Autodesk Inventor part; units mm, degrees
ref_plane "YZ Plane" through (0, 0, 0) normal (1, 0, 0) x (0, 1, 0)
ref_plane "XZ Plane" through (0, 0, 0) normal (0, 1, 0) x (-1, 0, 0)
ref_plane "XY Plane" through (0, 0, 0) normal (0, 0, 1) x (1, 0, 0)
sketch "Sketch1" plane through (0, 0, 0) normal (0, 0, 1) x (1, 0, 0)
  line L0 (-26.0453, 15.4617) -> (23.9547, 15.4617)
  line L1 (23.9547, 15.4617) -> (23.9547, -18.5383)
  line L2 (23.9547, -18.5383) -> (-26.0453, -18.5383)
  line L3 (-26.0453, -18.5383) -> (-26.0453, 15.4617)
  point P0 (0, 0)
  dimension "d0" = 50
  dimension "d1" = 34
extrude "Extrusion1" add sketch "Sketch1" along normal blind 2
sketch "Sketch2" plane through (0, 0, 2) normal (0, 0, 1) x (1, 0, 0)
  line L0 (-26.0453, 15.4617) -> (-26.0453, -18.5383)
  line L1 (23.9547, 15.4617) -> (-26.0453, 15.4617)
  point P0 (0, 0)
  point P1 (-23.0453, 11.4617)
  point P2 (-23.0453, -11.5383)
  point P3 (-13.0453, -16.5383)
  dimension "d4" = 23
  dimension "d5" = 3
  dimension "d6" = 3
  dimension "d7" = 4
  dimension "d8" = 5
  dimension "d9" = 10
hole "Hole1" at (-23.0453, 11.4617, 2) at (-23.0453, -11.5383, 2) at (-13.0453, -16.5383, 2) direction (0, 0, -1) diameter 2 depth 6.5 tip angle 118
sketch "Sketch3" plane through (0, 0, 2) normal (0, 0, 1) x (1, 0, 0)
  line L0 (-26.0453, 15.4617) -> (-26.0453, -18.5383)
  line L1 (-26.0453, 8.4617) -> (-23.0453, 8.4617)
  line L2 (-23.0453, 8.4617) -> (-23.0453, -7.5383)
  line L3 (-23.0453, -7.5383) -> (-26.0453, -7.5383)
  line L4 (-26.0453, -7.5383) -> (-26.0453, 8.4617)
  line L5 (23.9547, 15.4617) -> (-26.0453, 15.4617)
  circle A0 centre (-23.0453, -11.5383) radius 1
  point P0 (0, 0)
  dimension "d17" = 7
  dimension "d18" = 4
  dimension "d19" = 3
extrude "Extrusion2" cut sketch "Sketch3" against normal blind 2 contours L1 L2 L3 L0
chamfer "Chamfer1" distance 3 angle 45 2 edges at (-26.0453, 8.4617, 1) (-26.0453, -7.5383, 1)
sketch "Sketch5" plane through (0, 0, 2) normal (0, 0, 1) x (1, 0, 0)
  line L0 (-20.0453, 14.9617) -> (23.9547, 14.9617)
  line L1 (23.9547, 14.9617) -> (23.9547, -13.0383)
  line L2 (23.9547, -13.0383) -> (-20.0453, -13.0383)
  line L3 (-20.0453, -13.0383) -> (-20.0453, 14.9617)
  line L4 (23.9547, 15.4617) -> (-26.0453, 15.4617)
  line L5 (-26.0453, -18.5383) -> (23.9547, -18.5383)
  line L6 (-23.0453, 8.4617) -> (-23.0453, -7.5383)
  line L7 (23.9547, -18.5383) -> (23.9547, 15.4617)
  circle A0 centre (-13.0453, -16.5383) radius 1
  point P0 (0, 0)
  dimension "d27" = 3
  dimension "d28" = 0
  dimension "d29" = 50
  dimension "d30" = 3.5
  dimension "d31" = 31.5
  dimension "d32" = 0.5
extrude "Extrusion3" cut sketch "Sketch5" against normal blind 0.4 contours L0 L1 L2 L3
sketch "Sketch8" plane through (0, 0, 2) normal (0, 0, 1) x (1, 0, 0)
  line L0 (-26.0453, -18.5383) -> (23.9547, -18.5383)
  line L1 (11.9547, -18.5383) -> (-1.0453, -18.5383)
  line L2 (-1.0453, -18.5383) -> (-1.0453, -44.5383)
  line L3 (-1.0453, -44.5383) -> (11.9547, -44.5383)
  line L4 (11.9547, -44.5383) -> (11.9547, -18.5383)
  line L5 (23.9547, -18.5383) -> (23.9547, 15.4617)
  circle A0 centre (-13.0453, -16.5383) radius 1
  line L6 (6.9547, -38.5383) -> (6.9547, -18.5383) construction
  line L7 (9.4547, -38.5383) -> (9.4547, -18.5383)
  line L8 (4.4547, -18.5383) -> (4.4547, -38.5383)
  arc A1 (4.4547, -38.5383) -> (9.4547, -38.5383) centre (6.9547, -38.5383) ccw
  arc A2 (9.4547, -18.5383) -> (4.4547, -18.5383) centre (6.9547, -18.5383) ccw
  circle A3 centre (6.9547, -38.5383) radius 1
  point P0 (0, 0)
  point P1 (23.9547, -13.0383)
  point P2 (6.9547, -28.5383)
  dimension "d48" = 12
  dimension "d49" = 25
  dimension "d50" = 20
  dimension "d51" = 22
  dimension "d52" = 6
  dimension "d53" = 5
  dimension "d54" = 2
extrude "Extrusion6" add sketch "Sketch8" against normal blind 2 contours L0 L7 A1 L8
fillet "Fillet1" radius 5 2 edges at (4.4547, -18.5383, 1) (9.4547, -18.5383, 1)
sketch "Sketch9" plane through (0, 0, 2) normal (0, 0, 1) x (1, 0, 0)
  circle A0 centre (-13.0453, -16.5383) radius 1
  circle A1 centre (6.9547, -38.5383) radius 1
  line L0 (-13.0453, -16.5383) -> (6.9547, -38.5383) construction
  line L1 (-14.8951, -18.22) -> (5.1049, -40.22)
  line L2 (8.8046, -36.8566) -> (-11.1954, -14.8566)
  arc A2 (-11.1954, -14.8566) -> (-14.8951, -18.22) centre (-13.0453, -16.5383) ccw
  arc A3 (5.1049, -40.22) -> (8.8046, -36.8566) centre (6.9547, -38.5383) ccw
  line L3 (-26.0453, -18.5383) -> (-0.5453, -18.5383)
  line L4 (-14.6058, -18.5383) -> (-7.8485, -18.5383)
  line L5 (4.4547, -23.5383) -> (4.4547, -38.5383)
  line L6 (4.4547, -32.0718) -> (4.4547, -38.5383)
  line L7 (4.4547, -38.5383) -> (6.7171, -41.027)
  arc A4 (4.4547, -38.5383) -> (9.4547, -38.5383) centre (6.9547, -38.5383) ccw
  point P0 (0, 0)
  point P1 (-3.0453, -27.5383)
extrude "Extrusion7" add sketch "Sketch9" against normal blind 2 contours L3 L2 L5 A4 L1
fillet "Fillet2" radius 1 2 edges at (-7.8485, -18.5383, 1) (4.4547, -32.0718, 1)
sketch "Sketch10" plane through (-26.0453, 15.4617, 0) normal (0, 1, 0) x (1, 0, 0)
  line L0 (50, 0) -> (50, -2)
  line L1 (0, 0) -> (0, -2)
  line L2 (50, -2) -> (0, -2)
  line L3 (0, -2) -> (0, 0)
  line L4 (0, 0) -> (50, 0)
  line L5 (50, 0) -> (50, -2)
  point P0 (26.0453, 0)
extrude "Extrusion8" add sketch "Sketch10" along normal blind 2
sketch "Sketch13" plane through (23.9547, -18.5383, 2) normal (1, 0, 0) x (0, 0, -1)
  line L0 (0, 0) -> (0, 5.5)
  line L1 (0.4, 5.5) -> (0.4, 33.5)
  line L2 (0.4, 5.5) -> (0, 5.5)
  line L3 (-1.6, 5.5) -> (0.4, 9.5)
  line L4 (0, 5.5) -> (0.4, 5.5)
  line L5 (-1.6, 5.5) -> (0.4, 5.5)
  line L6 (0.4, 5.5) -> (0.4, 9.5)
  point P0 (2, 18.5383)
  point P1 (0.4, 30.4)
  dimension "d70" = 1.6
  dimension "d71" = 4
extrude "Extrusion11" add sketch "Sketch13" against normal blind 44
sketch "Sketch14" plane through (23.9547, -18.5383, 2) normal (1, 0, 0) x (0, 0, -1)
  line L0 (0, 33.5) -> (0, 36)
  line L1 (0.4, 33.5) -> (0.4, 9.5)
  line L2 (0, 33.5) -> (0.4, 33.5)
  line L3 (-1.6, 33.5) -> (0.4, 29.5)
  line L4 (-1.6, 33.5) -> (0.4, 33.5)
  line L5 (0.4, 29.5) -> (0.4, 33.5)
  point P0 (2, 18.5383)
  dimension "d74" = 1.6
  dimension "d75" = 4
extrude "Extrusion12" add sketch "Sketch14" against normal blind 44
sketch "Sketch15" plane through (0, 0, 0) normal (0, 0, -1) x (-1, 0, 0)
  line L0 (-23.9547, -18.5383) -> (-23.9547, 17.4617)
  line L1 (-23.9547, 17.4617) -> (-30.4547, 17.4617)
  line L2 (-30.4547, 17.4617) -> (-30.4547, -13.3383)
  line L3 (-30.4547, -13.3383) -> (-23.9547, -13.3383)
  line L4 (-23.9547, -13.3383) -> (-23.9547, 17.4617)
  line L5 (-14.4547, -18.5383) -> (-23.9547, -18.5383)
  point P0 (0, 0)
  dimension "d78" = 5.2
  dimension "d79" = 6.5
extrude "Extrusion13" add sketch "Sketch15" against normal blind 2
sketch "Sketch16" plane through (0, 0, 2) normal (0, 0, 1) x (1, 0, 0)
  line L0 (30.4547, -13.3383) -> (30.4547, 17.4617)
  line L1 (-20.0453, -9.0383) -> (23.9547, -9.0383)
  line L2 (30.4547, 10.9617) -> (-20.0453, 10.9617)
  line L3 (-20.0453, 10.9617) -> (-20.0453, -9.0383)
  line L4 (-20.0453, -9.0383) -> (30.4547, -9.0383)
  line L5 (30.4547, -9.0383) -> (30.4547, 10.9617)
  line L6 (23.9547, 10.9617) -> (-20.0453, 10.9617)
  point P0 (0, 0)
  point P1 (30.4547, -9.0383)
extrude "Extrusion14" cut sketch "Sketch16" against normal blind 0.4
Geometry: final body of the model. Coordinates: model frame, mm. A direction names the side the tool comes from. Round coordinates to 2 decimals unless told otherwise and drop trailing zeros. Order: outer loops, then holes, each group sorted by start corner. A loop starts at its lowest first (then second) coordinate and runs counter-clockwise, first axis right, second up. Notation, with made-up numbers: (-6.75, 17.5) -> (18.25, 17.5) arc R14 ccw to (18.25, 22.5) -> close; hole circle Ø11 at (8.25, -12.5). An arc over 180 degrees is marked (long way). Write each question's results on one line, items separated by ' | '.
Q1. Section query B-B (y = -21). Output: boundary loops of the cut face in (x, z), and give its area (3 significant figures).
Response values:
outline: (-12.37, 0) -> (-5.61, 0) -> (-5.61, 2) -> (-12.37, 2) -> close; (3.76, 0) -> (10.15, 0) -> (10.15, 2) -> (3.76, 2) -> close | area: 26.3 mm²
Q2. Section query C-C (x = -3). Output: boundary loops of the cut face in (y, z), and give its area (3 significant figures).
Response values:
outline: (-31.3, 0) -> (-23.87, 0) -> (-23.87, 2) -> (-31.3, 2) -> close; (-18.54, 0) -> (17.46, 0) -> (17.46, 2) -> (14.96, 2) -> (14.96, 3.6) -> (10.96, 1.6) -> (-9.04, 1.6) -> (-13.04, 3.6) -> (-13.04, 2) -> (-18.54, 2) -> close | area: 83.7 mm²
Q3. Ray query, line 1 along X through (y, z) = (-3.5, 0.9); line 2 along Z through (x, y) = (22, 8.5); line 3 along X through (y, z) = (-18, 1.55). Return the intervals inside material, ascending.
Response values:
line 1: -23.05 to 30.45 | line 2: 0 to 1.6 | line 3: -26.05 to 23.95
Q4. Section query A-A (x = 23). Output: boundary loops of the cut face in (y, z), and give its area (3 significant figures).
Response values:
outline: (-18.54, 0) -> (17.46, 0) -> (17.46, 2) -> (14.96, 2) -> (14.96, 3.6) -> (10.96, 1.6) -> (-9.04, 1.6) -> (-13.04, 3.6) -> (-13.04, 2) -> (-18.54, 2) -> close | area: 68.8 mm²
Q5. Pull-direction query (X, two-part tool) for faces 1 (the face through (27, -13.338, 1)), 2 (the face through (-3, -18.538, 1)), 3 (the face through (-20.045, 14.1, 2.5)); classes: released by +X, released by -X, zero draft, split by the parting line, or undercut.
Response values:
face 1: zero draft | face 2: undercut | face 3: released by -X
Q6. Section query D-D (y = 6). Output: boundary loops of the cut face in (x, z), and give its area (3 significant figures).
Response values:
outline: (-23.05, 0) -> (30.45, 0) -> (30.45, 1.6) -> (-20.05, 1.6) -> (-20.05, 2) -> (-23.05, 2) -> close | area: 86.8 mm²
Q7. Access query for faces 4 (the face through (5, 1, 1.6)), 5 (the face through (-20, -18.538, 1)), 6 (the face through (-20.045, -12.1, 2.5)), 7 (the face through (23.955, 14.1, 2.5)), 8 (the face through (-6.51, -19.15, 0.99)). Directions: +Z, -Z, +X, -X, +Y, -Y. A direction counts if a zero-diameter tool reaches every point of the face in a straight line with its end or side. Return the directions, or none.
Response values:
face 4: +Z, +X | face 5: +Z, -Z, -X, -Y | face 6: +Z, -X, +Y, -Y | face 7: +Z, +X, +Y, -Y | face 8: +Z, -Z
Q8. Pin query (flat end, axial travel): pin 1 Ø0.6 at (y, z) = (-26, 0.5) entering from -X; pin 2 Ø0.6 at (x, z) = (-21.5, 1) entering from -Y; pin 3 Ø17 at (x, y) = (-3, -24.5) entering from +Z; pin 4 Ø2.5 at (x, y) = (6.95, -38.54) entering from -Z. Return the tip coordinate at first contact, or that it passes through.
Response values:
pin 1: x = -8.1 | pin 2: y = -18.54 | pin 3: z = 2 | pin 4: z = 0
